Can you work these out from the model? Positions are in its coordinate system, mm. Round coordinates to 2 decimals unless told otherwise and drop trailing zeros. Write each loop counter-clockwise with the first axis right and the second up, starting at its lowest first coordinate (ties: lowest second). Pieces come first, ordered by that corner, then holes. Notation, with made-up numbers: M 35.5,48 L 62.5,48 A16 cw 62.5,63 Z; hole C -13,30 d8. An arc over 180 degrees is marked long. Answer in a Markdown table with one row per item. Add a question column.
(1) Suppose I cut it at A-A, the plane x = 0. Write out the boundary of the cut face in (y, z), then the cut area to 3 significant figures.
(2) If I drill on probe 1 along X at (y, z) = (2.5, 4.75); probe 2 along X at (y, z) = (2.1, 1.25); probe 3 along Z at (x, y) = (4.5, 3.25), over which ranges is the centre line in solid material (lowest first)?
(3) If we mould it in two halves opening along Z, with no side actions, what happens to faces 1 (the face through (5, 4, 5)), 2 (the face through (4, 2, 4)), 3 (the face through (-2.29, 3.81, 10.32))? For each: released by +Z, released by -Z, zero draft, split by the parting line, or undercut.
(4) Suppose I cut it at B-B, the plane y = 3.6. Write out the boundary of the cut face in (x, z).
(5) Suppose I cut it at C-C, the plane y = 1.2. Write out the boundary of the cut face in (x, z).
(6) I'm going to push flat-ended pins straight in: pin 1 (1 mm diameter, centred on y = 2, z = -2, fed in from -X); pin 2 (1 mm diameter, centred on y = 1.5, z = -5, fed in from +X); pin 3 (8.5 mm diameter, centred on x = 0, z = 0, fed in from -Y); pin 4 (4 mm diameter, centred on x = 5, z = -1, fed in from -Y). Where does each tip first touch, or does it pass through?
from build123d import *

# Parameters (mm, degrees)
SKETCH_1_R          = 12
SKETCH_2_R          = 10.5
SHELL_2_T           = -2
SKETCH_3_R          = 5.4
CUT_EXTRUDE_2_DEPTH = 18.435595935


with BuildPart() as part:
    # 草图1 → 放样1 section 0
    with BuildSketch(Plane(origin=(0, 0, 0), x_dir=(1, 0, 0), z_dir=(0, 1, 0))):
        Circle(SKETCH_1_R)
    # 草图2 → 放样1 section 1
    with BuildSketch(Plane(origin=(0, 4, 0), x_dir=(1, 0, 0), z_dir=(0, 1, 0))):
        Circle(SKETCH_2_R)
    loft()

    # 抽壳2
    shell_2_openings = [part.faces().sort_by_distance(p)[0] for p in [
        (0, 0, 0),
    ]]
    offset(amount=SHELL_2_T, openings=shell_2_openings, kind=Kind.INTERSECTION)

    # 草图3 → 切除-拉伸2 (cut, through all)
    with BuildSketch(Plane(origin=(0, 4, 0), x_dir=(1, 0, 0), z_dir=(0, 1, 0))):
        with Locations(Location((0, 0, 0), (0, 0, 270))):
            Circle(SKETCH_3_R)
    extrude(amount=-CUT_EXTRUDE_2_DEPTH, mode=Mode.SUBTRACT)


solid = part.part
Calculated:
| question | item | result |
|---|---|---|
| 1 | outline | M 0,-12 L 4,-10.5 L 4,-5.4 L 2,-5.4 L 2,-9.11 L 0,-9.86 Z; M 0,9.86 L 2,9.11 L 2,5.4 L 4,5.4 L 4,10.5 L 0,12 Z |
| 1 | area | 30.4 mm² |
| 2 | probe 1 | -9.99 to -2.57, 2.57 to 9.99 |
| 2 | probe 2 | -11.14 to -5.25, 5.25 to 11.14 |
| 2 | probe 3 | -9.8 to -2.98, 2.98 to 9.8 |
| 3 | face 1 | zero draft |
| 3 | face 2 | undercut |
| 3 | face 3 | split by the parting line |
| 4 | outline | C 0,0 d21.3; hole C 0,0 d10.8 |
| 5 | outline | C 0,0 d23.1; hole C 0,0 d18.83 |
| 6 | pin 1 | x = -11.28 |
| 6 | pin 2 | x = 10.6 |
| 6 | pin 3 | through |
| 6 | pin 4 | y = 2 |
